```python
from build123d import *

# Parameters (mm, degrees)
PAD_DEPTH   = 3
FILLET_R    = 1
FILLET001_R = 0.2
FILLET002_R = 1


with BuildPart() as part:
    # Sketch → Pad (new body)
    with BuildSketch(Plane.YZ):
        with BuildLine():
            ThreePointArc((4.330127, -2.5), (0, 5), (-4.330127, -2.5))
            Line((-4.330127, -2.5), (-4.330127, -5))
            Line((-4.330127, -5), (-5.428204, -6.499999))
            Line((-6.928204, -6.499999), (-5.428204, -6.499999))
            Line((-6.928204, -3.999999), (-6.928204, -6.499999))
            ThreePointArc((6.928204, -3.999999), (0, 8), (-6.928204, -3.999999))
            Line((6.928204, -3.999999), (6.928204, -6.499999))
            Line((6.928204, -6.499999), (5.428204, -6.499999))
            Line((4.330127, -5), (5.428204, -6.499999))
            Line((4.330127, -2.5), (4.330127, -5))
        make_face()
    extrude(amount=PAD_DEPTH)

    # Fillet
    fillet_edges = [part.edges().sort_by_distance(p)[0] for p in [
        (3, -6.928204, -5.249999),
        (3, 0, 8),
        (3, 6.928204, -5.249999),
    ]]
    fillet(fillet_edges, radius=FILLET_R)

    # Fillet001
    fillet001_edges = [part.edges().sort_by_distance(p)[0] for p in [
        (3, 0, 5),
        (3, -4.330127, -3.75),
        (3, -4.879165, -5.749999),
        (3, 4.330127, -3.75),
        (3, 4.879165, -5.749999),
    ]]
    fillet(fillet001_edges, radius=FILLET001_R)

    # Fillet002
    fillet002_edges = [part.edges().sort_by_distance(p)[0] for p in [
        (0, 0, 8),
        (0, 6.928204, -5.249999),
        (0, 4.330127, -3.75),
        (0, 0, 5),
        (0, -4.330127, -3.75),
        (0, -6.928204, -5.249999),
    ]]
    fillet(fillet002_edges, radius=FILLET002_R)


solid = part.part
```
The listing builds one solid part. Answer for the finished solid, in the listing's coordinates (mm). A direction names the side the tool comes from. Coordinates: 2 decimals unless noted, no trailing zeros. Loops run counter-clockwise (first coordinate to the right, second up) from the corner with the lowest first, then second, coordinate; pieces in that order, holes last. Notation, with made-up numbers: (-20, 69.25) - (27, 69.25) arc R12 cw to (27, 83.25) - close; hole circle Ø3 at (75, 63.25). An arc over 180 degrees is marked (long way). Write item = value, one per line.
1) Each of these flat-tipped pins is pushed along its axis until it touches: P1, Ø0.9, axis at x = 2, z = -3.5, coming from the -Y side; P2, Ø1.5, axis at x = 2.5, z = 1, coming from the +Y side; P3, Ø0.9, axis at x = 2, z = -4, coming from the +Y side. Where does it stop, or does it pass through?
Responses:
P1 = -7.4
P2 = 7.99
P3 = 7.17
2) Section B-B (x = 1.75) is taken. Determine the outline of the cut face in (y, z).
Responses:
outline = (-6.93, -6.5) - (-5.43, -6.5) - (-4.33, -5) - (-4.33, -2.5) arc R5 cw (long way) to (4.33, -2.5) - (4.33, -5) - (5.43, -6.5) - (6.93, -6.5) - (6.93, -4) arc R8 ccw (long way) to (-6.93, -4) - close
3) Find the intervals of material crossed by line 1 along Y through (x, z) = (1.65, 0); line 2 along Z through (x, y) = (1.4, 0); line 3 along Y through (x, z) = (0.3, 1), in increasing order.
Responses:
line_1 = -8 to -5, 5 to 8
line_2 = 5 to 8
line_3 = -7.65 to -5.19, 5.19 to 7.65
4) Determine the mould class of faces 5 (the face through (2.943, 4.979, -5.785)), 6 (the face through (2.7, 6.64, -5.13)), 7 (the face through (0, 2, 6)), 8 (the face through (2, -4.33, -4)) for opening direction Y: pulls with the +Y half, pulls with the -Y half, needs draft (parallel to the pull), parting line crosses it, or undercut.
Responses:
face_5 = undercut
face_6 = pulls with the +Y half
face_7 = needs draft
face_8 = undercut
5) Section D-D (x = 0.8) is taken. Determine the outline of the cut face in (y, z).
Responses:
outline = (-6.91, -6.5) - (-5.43, -6.5) - (-4.35, -5.03) - (-4.35, -2.51) arc R5.02 cw (long way) to (4.35, -2.51) - (4.35, -5.03) - (5.43, -6.5) - (6.91, -6.5) - (6.91, -3.99) arc R7.98 ccw (long way) to (-6.91, -3.99) - close
6) Section A-A (z = -4.5) is taken. Determine the outline of the cut face in (x, y).
Responses:
outline = (0, -5.93) arc R1 ccw to (1, -6.93) - (2, -6.93) arc R1 ccw to (3, -5.93) - (3, -4.53) arc R0.2 ccw to (2.8, -4.33) - (1, -4.33) arc R1 ccw to (0, -5.33) - close; (0, 5.33) arc R1 ccw to (1, 4.33) - (2.8, 4.33) arc R0.2 ccw to (3, 4.53) - (3, 5.93) arc R1 ccw to (2, 6.93) - (1, 6.93) arc R1 ccw to (0, 5.93) - close
7) Section C-C (y = 0) is taken. Determine the outline of the cut face in (x, z).
Responses:
outline = (0, 6) arc R1 ccw to (1, 5) - (2.8, 5) arc R0.2 ccw to (3, 5.2) - (3, 7) arc R1 ccw to (2, 8) - (1, 8) arc R1 ccw to (0, 7) - close
8) Which of the six approach directions +Z, -Z, +X, -X, +Y, -Y give full straight-line access (tool end or side, diameter ignored) to faces 1 (the face through (2.7, -6.64, -5.13)), 2 (the face through (0.3, -6.64, -5.13)), 3 (the face through (1.5, 6.928, -5.2)), 4 (the face through (2, 4.33, -4))?
Responses:
face_1 = -Z, +X, -Y
face_2 = -Z, -X, -Y
face_3 = -Z, +X, -X, +Y
face_4 = -Z, +X, -X
